Geometry check sheet. Reference: drawing and pictorial views, mm from the part's lowest x, y, z. Round coordinates to 2 decimals unless told otherwise and drop trailing zeros. Write each loop counter-clockwise with the first axis right and the second up, starting at its lowest first coordinate (ties: lowest second). Pieces come first, ordered by that corner, then holes. Notation, with made-up numbers: (4.25, 2) - (47.25, 2) arc R20 cw to (47.25, 28) - close; hole circle Ø1 at (43.5, 22.5). An arc over 180 degrees is marked (long way). Use one line per item in the form item = value. Start each with the question number.
1) Section check B-B (z = 2.25). Record the boundary of the cut face in (x, y) (1 decimal).
2) Section check A-A (x = 2). Record the boundary of the cut face in (y, z) (1 decimal).
3) Section check C-C (y = 9). Record the boundary of the cut face in (x, z) (1 decimal).
4) Gauge pin test, flat end, axial feed: P1, Ø1.5, axis at x = 2, y = 3, coming from the +Z side (1 decimal). Record the tip position at first contact, or that the pin passes through.
5) Scan lines: probe 1 along Y at (x, z) = (2.25, 12.25) (1 decimal); probe 2 along Z at (x, y) = (2.75, 4.75) (1 decimal). Record each from-to range of solid material in increasing order.
6) Draft check along Y on the marked faces 1, 2, 3 and 4. Enter one of: +Y half, -Y half, draft (parallel to the pull), parting line (faces both ways), or undercut.
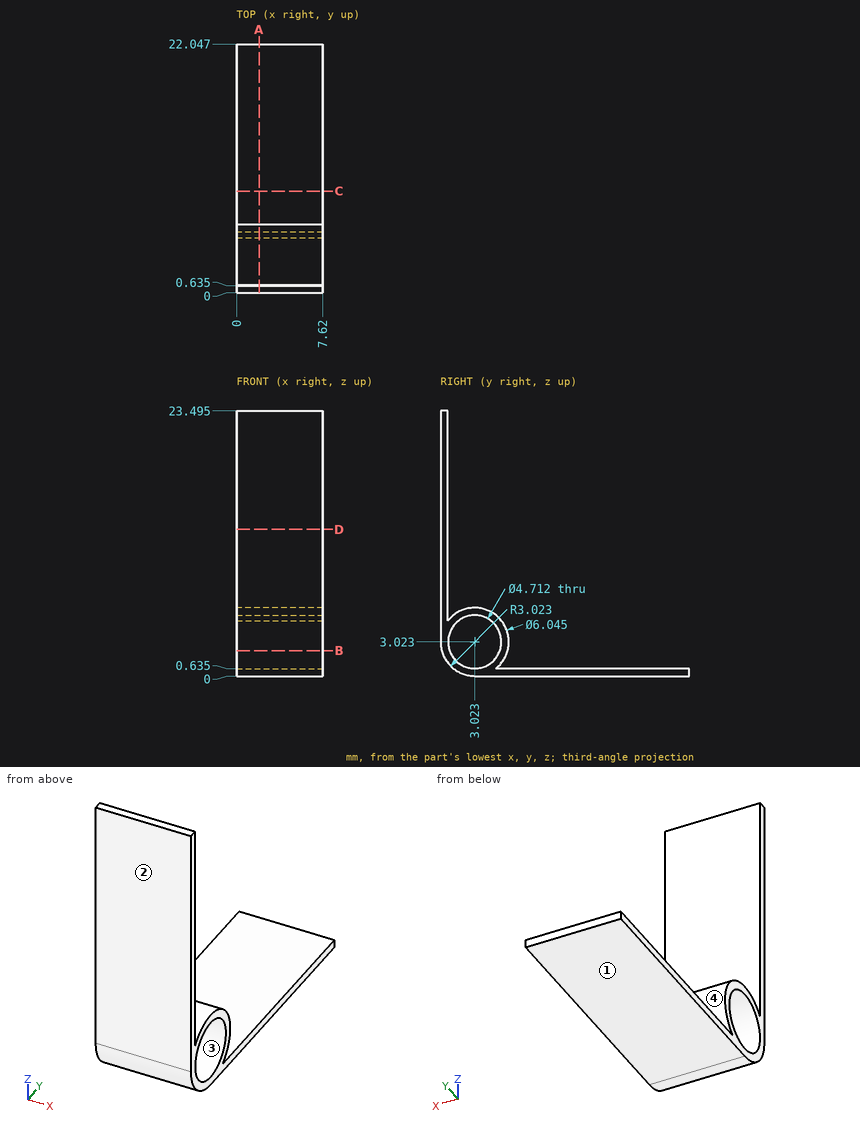
Results are:
q1.outline = (0, 0.1) - (7.6, 0.1) - (7.6, 0.8) - (0, 0.8) - close; (0, 5.2) - (7.6, 5.2) - (7.6, 5.9) - (0, 5.9) - close
q2.outline = (0, 3) arc R3 ccw to (3, 0) - (22, 0) - (22, 0.6) - (4.9, 0.6) arc R3 ccw (long way) to (0.6, 4.9) - (0.6, 23.5) - (0, 23.5) - close; hole circle Ø4.7 at (3, 3)
q3.outline = (0, 0) - (7.6, 0) - (7.6, 0.6) - (0, 0.6) - close
q4.P1 = 6
q5.probe_1 = 0 to 0.6
q5.probe_2 = 0 to 1.4, 4.6 to 5.5
q6.face_1 = draft
q6.face_2 = -Y half
q6.face_3 = undercut
q6.face_4 = undercut
